Could you check a few things on this model? Use its own coordinates, in mm. Face numbers are marked on the shaded views. A direction names the side the tool comes from. Coordinates: 2 decimals unless noted, no trailing zeros. Loops run counter-clockwise (first coordinate to the right, second up) from the corner with the lowest first, then second, coordinate; pieces in that order, holes last. Notation, with made-up numbers: (82, -20) -> (103, -20) arc R14 cw to (103, -8) -> close; hole circle Ø5 at (63, -2). An arc over 180 degrees is marked (long way). One line per question, with ' | ' between items. Start each with the question number.
(1) If we mould it in two halves opening along Z, with no side actions, what happens to the marked faces 4, 5 and 6? For each: pulls with the +Z half, pulls with the -Z half, needs draft (parallel to the pull), parting line crosses it, or undercut.
(2) Suppose I cut it at A-A (z = -5.5). Please give me the cut outline in (x, y).
(3) Which directions (+Z, -Z, +X, -X, +Y, -Y) give clear straight access to the entire face, cutting with the end or side of a thin tool? Please do the marked faces 1, 2 and 3.
(4) Suppose I cut it at B-B (y = -27). Please give me the cut outline in (x, z).
(5) Suppose I cut it at D-D (z = -28). Please give me the cut outline in (x, y).
(6) I'm going to push flat-ended pins straight in: pin 1 Ø4 at (y, z) = (-14, -3) entering from +X; pin 2 Ø12 at (x, y) = (-5.5, 0) entering from -Z; pin 3 Ø19 at (x, z) = (15, -29) entering from +Y. Where does each tip first touch, or does it pass through?
(7) If I drill on line 1 along X through (y, z) = (-44, -29); line 2 along Y through (x, z) = (-19, -16.5); line 3 along Z through (x, y) = (-20.5, -1), over which ranges is the centre line in solid material (lowest first)?
```python
from build123d import *

# Parameters (mm, degrees)
SKETCH1_R            = 6
BOSS_EXTRUDE1_DEPTH  = 10
BOSS_EXTRUDE3_START  = 5
SKETCH2_R            = 16
SKETCH2_R_2          = 6
BOSS_EXTRUDE3_DEPTH  = 5
SKETCH3_W            = 74
SKETCH3_H            = 5
BOSS_EXTRUDE5_DEPTH  = 5
FILLET4_R            = 5
SKETCH5_W            = 74
SKETCH5_H            = 10
BOSS_EXTRUDE8_DEPTH  = 31
BOSS_EXTRUDE10_DEPTH = 40
CUT_EXTRUDE1_DEPTH   = 10
FILLET5_R            = 5
FILLET6_R            = 5
FILLET7_R            = 12
FILLET8_R            = 12
SKETCH16_R           = 6
CUT_EXTRUDE2_DEPTH   = 10
SKETCH17_R           = 6
CUT_EXTRUDE3_DEPTH   = 10


with BuildPart() as part:
    # Sketch1 → Boss-Extrude1 (new body)
    with BuildSketch(Plane.XY):
        with BuildLine():
            Line((-47.000970423, -51.805827164), (26.999029577, -51.805827164))
            Line((26.999029577, -51.805827164), (26.999029577, -41.805827164))
            Line((26.999029577, -41.805827164), (21.633436879, -41.805827164))
            ThreePointArc((21.633436879, -41.805827164), (10.31972838, -37.119535663), (5.633436879, -25.805827164))
            Line((5.633436879, -25.805827164), (5.633436879, 10.194172836))
            ThreePointArc((5.633436879, 10.194172836), (-10.366563121, 26.194172836), (-26.366563121, 10.194172836))
            Line((-26.366563121, 10.194172836), (-26.366563121, -25.805827164))
            ThreePointArc((-26.366563121, -25.805827164), (-31.052854622, -37.119535663), (-42.366563121, -41.805827164))
            Line((-42.366563121, -41.805827164), (-47.000970423, -41.805827164))
            Line((-47.000970423, -41.805827164), (-47.000970423, -51.805827164))
        make_face()
        with Locations((-10.366563121, 10.194172836)):
            Circle(SKETCH1_R, mode=Mode.SUBTRACT)
    extrude(amount=-BOSS_EXTRUDE1_DEPTH)

    # Sketch2 → Boss-Extrude3 (add)
    with BuildSketch(Plane.XY.offset(BOSS_EXTRUDE3_START)):
        with Locations((-10.366563121, 10.194172836)):
            Circle(SKETCH2_R)
        with Locations((-10.366563121, 10.194172836)):
            Circle(SKETCH2_R_2, mode=Mode.SUBTRACT)
    extrude(amount=-BOSS_EXTRUDE3_DEPTH)

    # Sketch3 → Boss-Extrude5 (add)
    with BuildSketch(Plane.XY):
        with Locations((-10.000970423, -49.305827164)):
            Rectangle(SKETCH3_W, SKETCH3_H)
    extrude(amount=BOSS_EXTRUDE5_DEPTH)

    # Fillet4
    fillet4_edges = [part.edges().sort_by_distance(p)[0] for p in [
        (-10.000970423, -46.805827164, 0),
    ]]
    fillet(fillet4_edges, radius=FILLET4_R - 0.0001)  # a hair under: the kernel refuses the full size

    # Sketch5 → Boss-Extrude8 (add)
    with BuildSketch(Plane(origin=(0, 0, -10), x_dir=(-1, 0, 0), z_dir=(0, 0, -1))):
        with Locations((10.000970423, -46.805827164)):
            Rectangle(SKETCH5_W, SKETCH5_H)
    extrude(amount=BOSS_EXTRUDE8_DEPTH)

    # Sketch13 → Boss-Extrude10 (add)
    with BuildSketch(Plane(origin=(0, -41.805827164, 0), x_dir=(1, 0, 0), z_dir=(0, 1, 0))):
        Polygon((-10.091769113, 41), (-15.091769113, 41), (-15.091769113, 10), (-5.091769113, 10), (-5.091769113, 41), align=None)
    extrude(amount=BOSS_EXTRUDE10_DEPTH)

    # Sketch14 → Cut-Extrude1 (cut)
    with BuildSketch(Plane.ZY.offset(15.091769113)):
        Polygon((-41, -41.805827164), (-10, -1.805827164), (-41, -1.805827164), align=None)
    extrude(amount=-CUT_EXTRUDE1_DEPTH, mode=Mode.SUBTRACT)

    # Fillet5
    fillet5_edges = [part.edges().sort_by_distance(p)[0] for p in [
        (-28.729166117, -41.805827164, -10),
    ]]
    fillet(fillet5_edges, radius=FILLET5_R)

    # Fillet6
    fillet6_edges = [part.edges().sort_by_distance(p)[0] for p in [
        (8.270833883, -41.805827164, -10),
    ]]
    fillet(fillet6_edges, radius=FILLET6_R)

    # Fillet7
    fillet7_edges = [part.edges().sort_by_distance(p)[0] for p in [
        (26.999029577, -46.805827164, -41),
    ]]
    fillet(fillet7_edges, radius=FILLET7_R)

    # Fillet8
    fillet8_edges = [part.edges().sort_by_distance(p)[0] for p in [
        (-47.000970423, -46.805827164, -41),
    ]]
    fillet(fillet8_edges, radius=FILLET8_R)

    # Sketch16 → Cut-Extrude2 (cut)
    with BuildSketch(Plane(origin=(0, -41.805827164, 0), x_dir=(1, 0, 0), z_dir=(0, 1, 0))):
        with Locations(Location((14.999029577, 29, 0), (0, 0, 270))):
            Circle(SKETCH16_R)
    extrude(amount=-CUT_EXTRUDE2_DEPTH, mode=Mode.SUBTRACT)

    # Sketch17 → Cut-Extrude3 (cut)
    with BuildSketch(Plane(origin=(0, -41.805827164, 0), x_dir=(1, 0, 0), z_dir=(0, 1, 0))):
        with Locations(Location((-35.000970423, 29, 0), (0, 0, 270))):
            Circle(SKETCH17_R)
    extrude(amount=-CUT_EXTRUDE3_DEPTH, mode=Mode.SUBTRACT)


solid = part.part
```
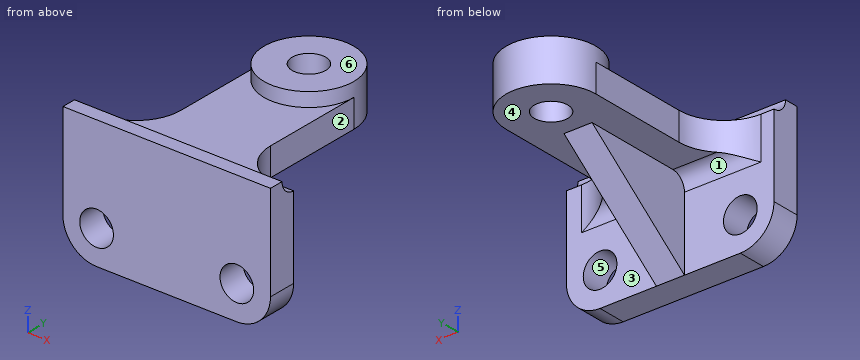
Checks:
1) face 4: pulls with the -Z half | face 5: undercut | face 6: pulls with the +Z half
2) outline: (-47, -51.81) -> (27, -51.81) -> (27, -41.81) -> (21.63, -41.81) arc R16 cw to (5.63, -25.81) -> (5.63, 10.19) arc R16 ccw to (-26.37, 10.19) -> (-26.37, -25.81) arc R16 cw to (-42.37, -41.81) -> (-47, -41.81) -> close; hole circle Ø12 at (-10.37, 10.19)
3) face 1: -Z, -X, +Y | face 2: +Z, -Z, +X, +Y | face 3: -Z, +X, +Y
4) outline: (-26.41, -10) -> (-15.09, -10) -> (-15.09, -29.53) -> (-5.09, -29.53) -> (-5.09, -10) -> (5.68, -10) -> (5.68, 0) -> (-26.41, 0) -> close
5) outline: (-47, -51.81) -> (-40.92, -51.81) -> (-40.92, -41.81) -> (-47, -41.81) -> close; (-29.08, -51.81) -> (9.08, -51.81) -> (9.08, -41.81) -> (-5.09, -41.81) -> (-5.09, -25.03) -> (-15.09, -25.03) -> (-15.09, -41.81) -> (-29.08, -41.81) -> close; (20.92, -51.81) -> (27, -51.81) -> (27, -41.81) -> (20.92, -41.81) -> close
6) pin 1: stops at x = 5.63 | pin 2: stops at z = -13.25 | pin 3: stops at y = -41.81
7) line 1: x = -47 to -41, -29 to 9, 21 to 27 | line 2: y = -51.81 to -41.81 | line 3: z = -10 to 5
